from build123d import *

# Parameters (mm, degrees)
F0_W     = 83
F0_H     = 49
F1_DEPTH = 1.6
F3_D     = 4
F4_D     = 9.6
F5_D     = 3.1


with BuildPart() as f1:
    # F0 (on Front) → F1 (new body)
    with BuildSketch(Plane.XZ):
        with Locations((0, -3.527498)):
            Rectangle(F0_W, F0_H)
    extrude(amount=-F1_DEPTH)

    # F3 (through all)
    with Locations(Plane.XZ):
        with Locations((-38, -3.527498), (38, -3.527498)):
            Hole(F3_D / 2)

    # F4 (through all)
    with Locations(Plane.XZ):
        with Locations((0, -3.527498)):
            Hole(F4_D / 2)

    # F5 (through all)
    with Locations(Plane.XZ):
        with Locations((4.75, -11.754739)):
            Hole(F5_D / 2)


solid = f1.part
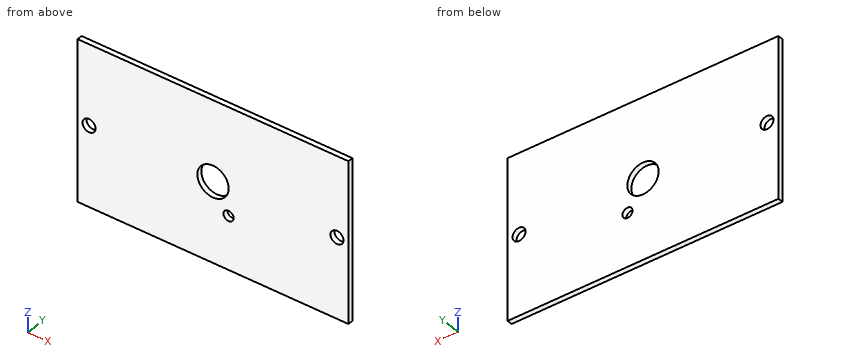
Check sheet for the modelled part. Datum: model origin and axes. Units: mm. Round coordinates to 2 decimals unless told otherwise and drop trailing zeros. Order: outer loops, then holes, each group sorted by start corner. A loop starts at its lowest first (then second) coordinate and runs counter-clockwise, first axis right, second up. Notation, with made-up numbers: M -33.5,35 L -23.5,35 A29 cw -23.5,61 Z; hole C -30,44.5 d10. An arc over 180 degrees is marked long. One line per item, written item: value. Start each with the question number.
1. Section check A-A on x = -38. Enter the section's corners in (y, z), and give its area (3 significant figures).
2. Section check B-B on z = 0. Enter the section's corners in (x, y), and give its area (3 significant figures).
3. Scan lines: line 1 along X through (y, z) = (1.4, -3.5); line 2 along Z through (x, y) = (0, 0.3); line 3 along Z through (x, y) = (3.5, 1.2). Record each from-to range of solid material in increasing order.
4. Gauge pin test, flat end, axial feed: P1, Ø8.5, axis at x = 0, z = -3.53, coming from the +Y side. Record the tip position at first contact, or that the pin passes through.
Results found:
1. outline: M 0,-28.03 L 1.6,-28.03 L 1.6,-5.53 L 0,-5.53 Z; M 0,-1.53 L 1.6,-1.53 L 1.6,20.97 L 0,20.97 Z
1. area: 72.0 mm^2
2. outline: M -41.5,0 L -3.26,0 L -3.26,1.6 L -41.5,1.6 Z; M 3.26,0 L 41.5,0 L 41.5,1.6 L 3.26,1.6 Z
2. area: 122 mm^2
3. line 1: -41.5 to -40, -36 to -4.8, 4.8 to 36, 40 to 41.5
3. line 2: -28.03 to -8.33, 1.27 to 20.97
3. line 3: -28.03 to -12.67, -10.84 to -6.81, -0.24 to 20.97
4. P1: through
